from build123d import *

# Parameters (mm, degrees)
BOSS_EXTRUDE1_DEPTH = 3
SKETCH2_R           = 1
CUT_EXTRUDE1_DEPTH  = 13


with BuildPart() as part:
    # Sketch1 → Boss-Extrude1 (new body)
    with BuildSketch(Plane(origin=(0, 0, 0), x_dir=(1, 0, 0), z_dir=(0, 1, 0))):
        with BuildLine():
            Line((-12.5, 0), (-25, 6))
            Line((-25, 6), (-25, 14))
            Line((-25, 14), (-12.5, 20))
            Line((-12.5, 20), (0, 20))
            Line((0, 20), (0, 15))
            Line((0, 15), (5, 15))
            ThreePointArc((5, 15), (23.660254038, 10), (5, 5))
            Line((5, 5), (0, 5))
            Line((0, 5), (0, 0))
            Line((0, 0), (-12.5, 0))
        make_face()
    extrude(amount=BOSS_EXTRUDE1_DEPTH)

    # Sketch2 → Cut-Extrude1 (cut)
    with BuildSketch(Plane(origin=(0, 3, 0), x_dir=(1, 0, 0), z_dir=(0, 1, 0))):
        with Locations(Location((13.660254038, 10, 0), (0, 0, 270))):
            Circle(SKETCH2_R)
    extrude(amount=-CUT_EXTRUDE1_DEPTH, mode=Mode.SUBTRACT)


solid = part.part
Input: part model. Units: mm. Frame: model coordinates. A direction names the side the tool comes from. Give positions to 0.01 mm unless a question says otherwise; leave off trailing zeros. Loops run counter-clockwise (first coordinate to the right, second up) from the corner with the lowest first, then second, coordinate; pieces in that order, holes last. Notation, with made-up numbers: (4.5, 5.5) -> (50.5, 5.5) arc R24 cw to (50.5, 33.5) -> close; hole circle Ø5 at (83, 81.5). An arc over 180 degrees is marked (long way). Answer as a JSON object with one key per item and string values. Group by question number.
Item 1: Cut plane B-B, the plane y = 2.1. Return the cut outline in (x, z).
Item 2: Cut plane C-C, the plane x = -14.5. Return the cut outline in (y, z), and give its area (3 significant figures).
Item 3: Pin query (flat end, axial travel): P1, Ø0.9, axis at x = 3, y = 2, coming from the +Z side; P2, Ø1.5, axis at x = 15.5, y = 1.5, coming from the +Z side; P3, Ø1, axis at y = 1, z = -15.5, coming from the -X side. Return the tip coordinate at first contact, or that it passes through.
Item 4: Pull-direction query (X, two-part tool) for faces 4 (the flat face through (0, 3, -10)), 5 (the cylindrical face through (13.05, 1.52, -10.79)), 6 (the flat face through (-18.662, 1.479, -2.958)); classes: released by +X, released by -X, zero draft, split by the parting line, or undercut.
Item 5: Reachability of faces 1 (the flat face through (0, 1, -18)), 2 (the flat face through (3, 1, -5)), 3 (the flat face through (-6, 1, 0)) from +Z, -Z, +X, -X, +Y, -Y: full face, straight path, thin tool, end or side. Return the list, or none.
Item 6: Line query: probe 1 along X at (y, z) = (1.35, -10); probe 2 along X at (y, z) = (0.6, -2.25); probe 3 along Z at (x, y) = (14, 1.3). Output: solid intervals per line, ascending.
Item 7: Cut plane A-A, the plane z = -10. Return the cut outline in (x, y), and give its area (3 significant figures).
Item 8: Cut plane D-D, the plane x = 9. Return the cut outline in (y, z).
Checks:
{
 "1": {"outline": "(-25, -14) -> (-12.5, -20) -> (0, -20) -> (0, -15) -> (5, -15) arc R10 ccw (long way) to (5, -5) -> (0, -5) -> (0, 0) -> (-12.5, 0) -> (-25, -6) -> close; hole circle Ø2 at (13.66, -10)"},
 "2": {"outline": "(0, -19.04) -> (3, -19.04) -> (3, -0.96) -> (0, -0.96) -> close", "area": "54.2 mm²"},
 "3": {"P1": "stops at z = -5", "P2": "stops at z = -0.06", "P3": "stops at x = -22.92"},
 "4": {"face 4": "zero draft", "face 5": "undercut", "face 6": "released by -X"},
 "5": {"face 1": "-Z, +Y, -Y", "face 2": "+Z, +Y, -Y", "face 3": "+Z, +X, -X, +Y, -Y"},
 "6": {"probe 1": "x = -25 to 12.66, 14.66 to 23.66", "probe 2": "x = -17.19 to 0, 7.34 to 19.98", "probe 3": "z = -19.99 to -10.94, -9.06 to -0.01"},
 "7": {"outline": "(-25, 0) -> (12.66, 0) -> (12.66, 3) -> (-25, 3) -> close; (14.66, 0) -> (23.66, 0) -> (23.66, 3) -> (14.66, 3) -> close", "area": "140 mm²"},
 "8": {"outline": "(0, -18.85) -> (3, -18.85) -> (3, -1.15) -> (0, -1.15) -> close"}
}
